Part model, mm, in its own coordinate system. Round coordinates to 2 decimals unless told otherwise and drop trailing zeros. Write each loop counter-clockwise with the first axis right and the second up, starting at its lowest first coordinate (ties: lowest second). Pieces come first, ordered by that corner, then holes.
from build123d import *

# Parameters (mm, degrees)
BOSS_EXTRUDE1_DEPTH = 300
SKETCH2_R           = 3
CUT_EXTRUDE1_DEPTH  = 4.5
SKETCH3_R           = 1.75
CUT_EXTRUDE2_DEPTH  = 301.166620396
CUT_EXTRUDE3_DEPTH  = 3
SKETCH5_W           = 12
SKETCH5_H           = 125
CUT_EXTRUDE5_DEPTH  = 301.101649446


with BuildPart() as part:
    # Sketch1 → Boss-Extrude1 (new body)
    with BuildSketch(Plane.XY):
        with BuildLine():
            Line((-5.6, 4), (5.6, 4))
            ThreePointArc((5.6, 4), (5.882842712, 3.882842712), (6, 3.6))
            Line((6, 3.6), (6, 2.8))
            Line((6, 2.8), (5.2, 2))
            Line((5.2, 2), (4.4, 2))
            Line((4.4, 2), (4.4, 1))
            Line((4.4, 1), (5.2, 1))
            Line((5.2, 1), (6, 0.2))
            Line((6, 0.2), (6, -3.6))
            ThreePointArc((6, -3.6), (5.882842712, -3.882842712), (5.6, -4))
            Line((5.6, -4), (-5.6, -4))
            ThreePointArc((-5.6, -4), (-5.882842712, -3.882842712), (-6, -3.6))
            Line((-6, -3.6), (-6, 0.2))
            Line((-6, 0.2), (-5.2, 1))
            Line((-5.2, 1), (-4.4, 1))
            Line((-4.4, 1), (-4.4, 2))
            Line((-4.4, 2), (-5.2, 2))
            Line((-5.2, 2), (-6, 2.8))
            Line((-6, 2.8), (-6, 3.6))
            ThreePointArc((-6, 3.6), (-5.882842712, 3.882842712), (-5.6, 4))
        make_face()
    extrude(amount=BOSS_EXTRUDE1_DEPTH)

    # Sketch2 → Cut-Extrude1 (cut)
    with BuildSketch(Plane(origin=(0, 4, 0), x_dir=(1, 0, 0), z_dir=(0, 1, 0))):
        with Locations(Location((0, -290, 0), (0, 0, 270))):
            Circle(SKETCH2_R)
        with Locations(Location((0, -265, 0), (0, 0, 270))):
            Circle(SKETCH2_R)
        with Locations(Location((0, -240, 0), (0, 0, 270))):
            Circle(SKETCH2_R)
        with Locations(Location((0, -215, 0), (0, 0, 270))):
            Circle(SKETCH2_R)
        with Locations(Location((0, -190, 0), (0, 0, 270))):
            Circle(SKETCH2_R)
        with Locations(Location((0, -165, 0), (0, 0, 270))):
            Circle(SKETCH2_R)
        with Locations(Location((0, -140, 0), (0, 0, 270))):
            Circle(SKETCH2_R)
        with Locations(Location((0, -115, 0), (0, 0, 270))):
            Circle(SKETCH2_R)
        with Locations(Location((0, -90, 0), (0, 0, 270))):
            Circle(SKETCH2_R)
        with Locations(Location((0, -65, 0), (0, 0, 270))):
            Circle(SKETCH2_R)
        with Locations(Location((0, -40, 0), (0, 0, 270))):
            Circle(SKETCH2_R)
        with Locations(Location((0, -15, 0), (0, 0, 270))):
            Circle(SKETCH2_R)
        with Locations((0, 10)):
            Circle(SKETCH2_R)
        with Locations((0, 35)):
            Circle(SKETCH2_R)
        with Locations((0, 60)):
            Circle(SKETCH2_R)
        with Locations((0, 85)):
            Circle(SKETCH2_R)
        with Locations((0, 110)):
            Circle(SKETCH2_R)
        with Locations((0, 135)):
            Circle(SKETCH2_R)
    extrude(amount=-CUT_EXTRUDE1_DEPTH, mode=Mode.SUBTRACT)

    # Sketch3 → Cut-Extrude2 (cut, through all)
    with BuildSketch(Plane(origin=(0, 4, 0), x_dir=(1, 0, 0), z_dir=(0, 1, 0))):
        with Locations(Location((0, -290.001504258, 0), (0, 0, 270))):
            Circle(SKETCH3_R)
        with Locations(Location((0, -265.001504258, 0), (0, 0, 270))):
            Circle(SKETCH3_R)
        with Locations(Location((0, -240.001504258, 0), (0, 0, 270))):
            Circle(SKETCH3_R)
        with Locations(Location((0, -215.001504258, 0), (0, 0, 270))):
            Circle(SKETCH3_R)
        with Locations(Location((0, -190.001504258, 0), (0, 0, 270))):
            Circle(SKETCH3_R)
        with Locations(Location((0, -165.001504258, 0), (0, 0, 270))):
            Circle(SKETCH3_R)
        with Locations(Location((0, -140.001504258, 0), (0, 0, 270))):
            Circle(SKETCH3_R)
        with Locations(Location((0, -115.001504258, 0), (0, 0, 270))):
            Circle(SKETCH3_R)
        with Locations(Location((0, -90.001504258, 0), (0, 0, 270))):
            Circle(SKETCH3_R)
        with Locations(Location((0, -65.001504258, 0), (0, 0, 270))):
            Circle(SKETCH3_R)
        with Locations(Location((0, -40.001504258, 0), (0, 0, 270))):
            Circle(SKETCH3_R)
        with Locations(Location((0, -15.001504258, 0), (0, 0, 270))):
            Circle(SKETCH3_R)
        with Locations((0, 9.998495742)):
            Circle(SKETCH3_R)
        with Locations((0, 34.998495742)):
            Circle(SKETCH3_R)
        with Locations((0, 59.998495742)):
            Circle(SKETCH3_R)
    extrude(amount=-CUT_EXTRUDE2_DEPTH, mode=Mode.SUBTRACT)

    # Sketch4 → Cut-Extrude3 (cut)
    with BuildSketch(Plane.XZ.offset(4)):
        Polygon((-6, 125), (-2, 125), (-2, 127), (-4, 127), (0, 133), (4, 127), (2, 127), (2, 125), (6, 125), (29.677261244, -70.087794046), (-63.472645217, -88.905956967), align=None)
    extrude(amount=-CUT_EXTRUDE3_DEPTH, mode=Mode.SUBTRACT)

    # Sketch5 → Cut-Extrude5 (cut, through all)
    with BuildSketch(Plane.XZ.offset(1)):
        with Locations((0, 62.5)):
            Rectangle(SKETCH5_W, SKETCH5_H)
    extrude(amount=-CUT_EXTRUDE5_DEPTH, mode=Mode.SUBTRACT)


solid = part.part
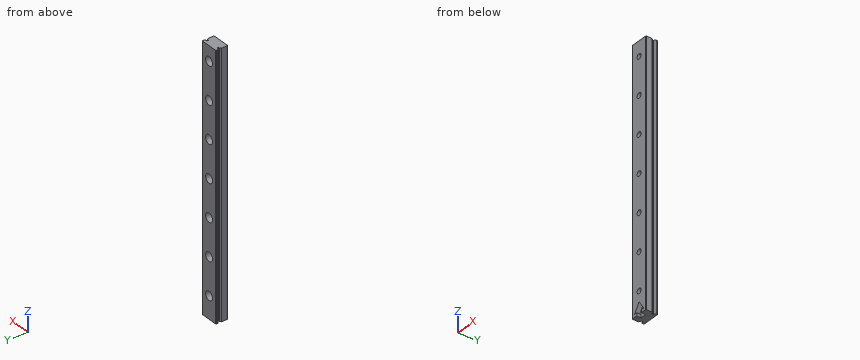
Q1. Wall check: line 1 (Y direction, x = 5, z = 249); line 2 (X direction, y = 1.75, z = 190); line 3 (X direction, y = -1.75, z = 140). Give the ranges that are in metal, low to high.
Q2. Saw through at A-A, the plane z = 290. Write the cut outline in (x, y), and give its area (3 significant figures).
Q3. Drop flat-ended pins along their axis: P1, Ø6.5, axis at x = -0.5, z = 290.5, coming from the +Y side; P2, Ø4, axis at x = 0, z = 215, coming from the +Y side; P3, Ø3, axis at x = 0, z = 190, coming from the -Y side. Give the stop position or say it passes through.
Computed:
1. line 1: y = -4 to 1, 2 to 4
1. line 2: x = -4.4 to -3, 3 to 4.4
1. line 3: x = -6 to -1.75, 1.75 to 6
2. outline: (-6, -3.6) arc R0.4 ccw to (-5.6, -4) - (-1.75, -4) - (-1.75, -0.5) - (-3, -0.5) - (-3, 4) - (-5.6, 4) arc R0.4 ccw to (-6, 3.6) - (-6, 2.8) - (-5.2, 2) - (-4.4, 2) - (-4.4, 1) - (-5.2, 1) - (-6, 0.2) - close; (1.75, -4) - (5.6, -4) arc R0.4 ccw to (6, -3.6) - (6, 0.2) - (5.2, 1) - (4.4, 1) - (4.4, 2) - (5.2, 2) - (6, 2.8) - (6, 3.6) arc R0.4 ccw to (5.6, 4) - (3, 4) - (3, -0.5) - (1.75, -0.5) - close
2. area: 52.1 mm2
3. P1: stops at y = 4
3. P2: stops at y = -0.5
3. P3: passes through
